from build123d import *

# Parameters (mm, degrees)
SKETCH1_R           = 13.5
SKETCH1_R_2         = 11.5
EXTRUDE_THIN2_DEPTH = 16
BOSS_EXTRUDE1_START = 2
SKETCH2_R           = 13.5
BOSS_EXTRUDE1_DEPTH = 2
SKETCH3_R           = 12.5
SKETCH3_R_2         = 11.5
EXTRUDE_THIN3_DEPTH = 4
CHAMFER1_SIZE       = 1
CHAMFER1_SIZE_2     = 4


with BuildPart() as part:
    # Sketch1 → Extrude-Thin2 (new body)
    with BuildSketch(Plane.XY):
        Circle(SKETCH1_R)
        Circle(SKETCH1_R_2, mode=Mode.SUBTRACT)
    extrude(amount=EXTRUDE_THIN2_DEPTH)

    # Sketch2 → Boss-Extrude1 (add)
    with BuildSketch(Plane(origin=(0, 0, 0), x_dir=(-1, 0, 0), z_dir=(0, 0, -1)).offset(BOSS_EXTRUDE1_START)):
        Circle(SKETCH2_R)
    extrude(amount=-BOSS_EXTRUDE1_DEPTH)

    # Sketch3 → Extrude-Thin3 (add)
    with BuildSketch(Plane.XY.offset(16)):
        Circle(SKETCH3_R)
        Circle(SKETCH3_R_2, mode=Mode.SUBTRACT)
    extrude(amount=EXTRUDE_THIN3_DEPTH)

    # Chamfer1
    # the kernel refuses this chamfer: 4, 1 mm, written as the material it adds along each edge
    with BuildSketch(Plane(origin=(0, 0, 16), x_dir=(1, 0, 0), z_dir=(0, -1, 0))) as chamfer1_piece_1_section:
        Polygon((12.5 + CHAMFER1_SIZE, 0), (12.5, CHAMFER1_SIZE_2), (12.5, 0), align=None)
    chamfer1_piece_1 = revolve(axis=Axis((0, 0, 16), (0, 0, 1)), mode=Mode.PRIVATE)
    chamfer1_piece_1 = chamfer1_piece_1 & Plane(origin=(0, 0, 17.985898728), x_dir=(1, 0, 0), z_dir=(0, 0, -1)) * Cylinder(13.5, 54, mode=Mode.PRIVATE)
    chamfer1_piece_1 = split(chamfer1_piece_1, bisect_by=Plane(origin=(-12.943594911, 0, 20), z_dir=(0, 0, -1)), keep=Keep.TOP, mode=Mode.PRIVATE)
    add(chamfer1_piece_1)


solid = part.part
Input: part model. Units: mm. Frame: model coordinates. Give positions to 0.01 mm unless a question says otherwise; leave off trailing zeros. Write each loop counter-clockwise with the first axis right and the second up, starting at its lowest first coordinate (ties: lowest second). Pieces come first, ordered by that corner, then holes.
Q1. Section C-C, the plane z = -0.5. Output: boundary loops of the cut face in (x, y).
Q2. First-contact query: P1, Ø12, axis at x = 9, z = 9, coming from the -Y side; P2, Ø6, axis at y = -2, z = 13.5, coming from the -X side; P3, Ø5, axis at y = 11, z = 14, coming from the +X side; P4, Ø2, axis at x = -8.5, y = -3, coming from the +Z side. Flat tips, straight axial feed; report the tip coordinate or a pass-through.
Q3. Section A-A, the plane x = 0. Output: boundary loops of the cut face in (y, z).
Q4. Material intervals for probe 1 along Y at (x, z) = (0, 5.5); probe 2 along X at (y, z) = (-8, 13), sorted ascending.
Q5. Pull-direction query (Y, two-part tool) for faces 1 (the face through (-2.72, -12.25, 19.81)), 2 (the face through (11, -4, 20)), 3 (the face through (0, 0, 0)); classes: pulls with the +Y half, pulls with the -Y half, needs draft (parallel to the pull), parting line crosses it, or undercut.
Q6. Section B-B, the plane z = 17. Output: boundary loops of the cut face in (x, y), plus the area to 3 significant figures.
Filled in:
1. outline: circle Ø27 at (0, 0)
2. P1: stops at y = -13.16
2. P2: stops at x = -13.5
2. P3: stops at x = 10.49
2. P4: stops at z = 0
3. outline: (-13.5, -2) - (13.5, -2) - (13.5, 16) - (12.5, 20) - (11.5, 20) - (11.5, 0) - (-11.5, 0) - (-11.5, 20) - (-12.5, 20) - (-13.5, 16) - close
4. probe 1: y = -13.5 to -11.5, 11.5 to 13.5
4. probe 2: x = -10.87 to -8.26, 8.26 to 10.87
5. face 1: parting line crosses it
5. face 2: needs draft
5. face 3: undercut
6. outline: circle Ø26.5 at (0, 0); hole circle Ø23 at (0, 0)
6. area: 136 mm2
